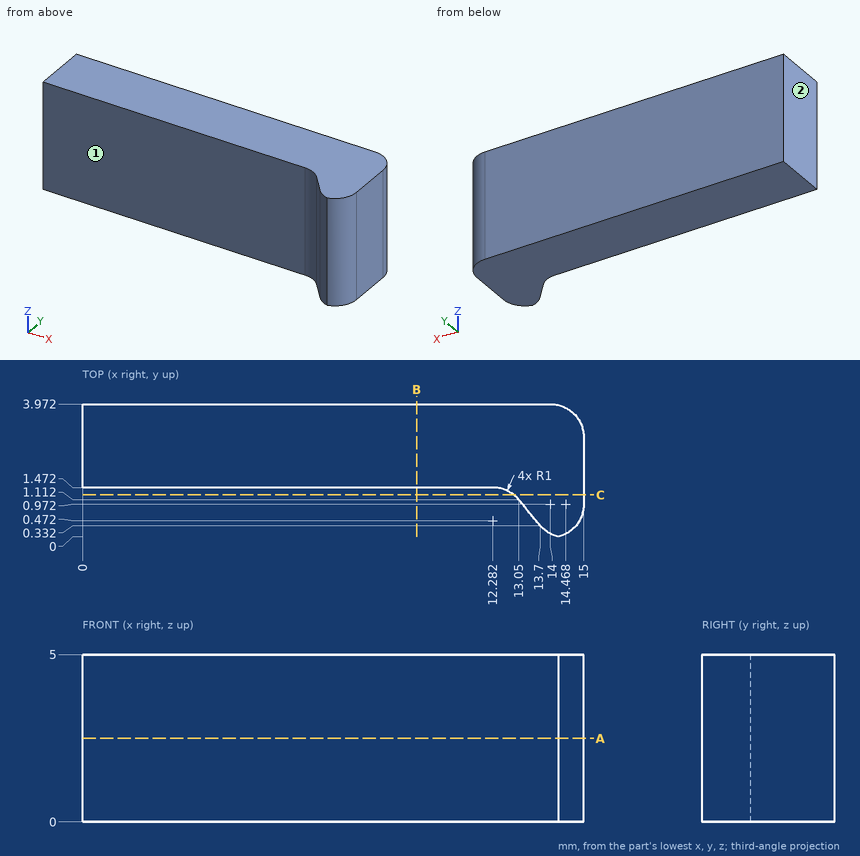
Part print with two shaded views. Sizes in mm from the minimum x, y, z corner. A direction names the side the tool comes from. Round coordinates to 2 decimals unless told otherwise and drop trailing zeros. Order: outer loops, then holes, each group sorted by start corner. A loop starts at its lowest first (then second) coordinate and runs counter-clockwise, first axis right, second up. Notation, with made-up numbers: (54.25, 36) - (82.25, 36) arc R11 cw to (82.25, 40) - close; hole circle Ø6 at (-3, -4). An arc over 180 degrees is marked (long way). Return JSON: item names as keys, results as strings.
(1) Pin check, flat tip, straight feed: pin 1 Ø1.5 at (x, z) = (9, 1.5) entering from -Y. Stop position of the tip, or through.
Answer key:
{"pin 1": "stops at y = 1.47"}
(2) Tool access for the marked faces 1 and 2: list every direction of +Z, -Z, +X, -X, +Y, -Y with a clear straight run to the whole face (end or side of a thin tool).
Answer key:
{"face 1": "+Z, -Z, -X, -Y", "face 2": "+Z, -Z, -X, +Y, -Y"}
(3) Cut at C-C (y = 1.25). Give the cut face in (x, z).
Answer key:
{"outline": "(12.91, 0) - (15, 0) - (15, 5) - (12.91, 5) - close"}
(4) Wall check: probe 1 along Y at (x, z) = (6.25, 1.2); probe 2 along X at (y, z) = (0.9, 1.35) (1 decimal); probe 3 along X at (y, z) = (3.45, 0.35). Give the ranges that are in metal, low to high. Write a range as from..to.
Answer key:
{"probe 1": "y = 1.47..3.97", "probe 2": "x = 13.2..15", "probe 3": "x = 0..14.88"}
(5) Cut at B-B (x = 10). Give the cut face in (y, z).
Answer key:
{"outline": "(1.47, 0) - (3.97, 0) - (3.97, 5) - (1.47, 5) - close"}
(6) Cut at A-A (z = 2.5). Give the cut face in (x, y), then the cut area to 3 significant figures.
Answer key:
{"outline": "(0, 1.47) - (12.28, 1.47) arc R1 cw to (13.05, 1.11) - (13.7, 0.33) arc R1 ccw to (14.23, 0) arc R1 ccw to (15, 0.97) - (15, 2.97) arc R1 ccw to (14, 3.97) - (0, 3.97) - close", "area": "39.5 mm^2"}
